Here's how the part is built. I have some questions about the finished solid (model axes, mm). Round coordinates to 2 decimals unless told otherwise and drop trailing zeros. Write each loop counter-clockwise with the first axis right and the second up, starting at its lowest first coordinate (ties: lowest second). Pieces come first, ordered by that corner, then holes. Notation, with made-up numbers: (32, 73.5) -> (38, 73.5) arc R24 cw to (38, 85.5) -> close; hole circle Ø6 at (55, -28.5). An arc over 180 degrees is marked (long way). Answer as CSV lines item,"result".
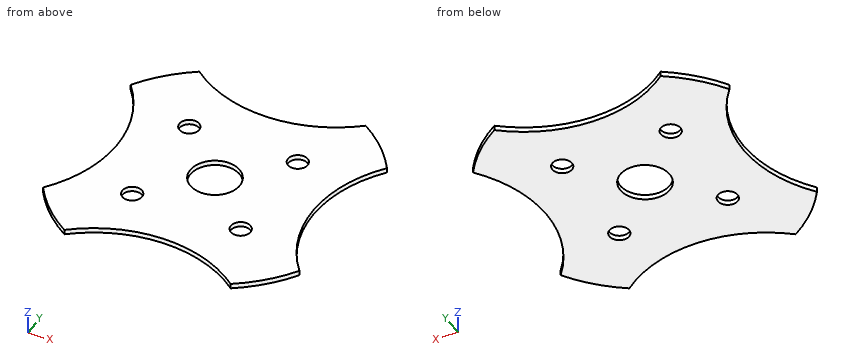
from build123d import *

# Parameters (mm, degrees)
EXTRUDE1_DEPTH     = 3.175
CUT_EXTRUDE1_REACH = 5.175
SKETCH2_R          = 6.35
SKETCH2_R_2        = 15.875


with BuildPart() as part:
    # Sketch1 → Extrude1 (new body)
    with BuildSketch(Plane.XY):
        with BuildLine():
            ThreePointArc((-53.553513238, 82.55), (0, 63.5), (53.553513238, 82.55))
            ThreePointArc((53.553513238, 82.55), (69.579024426, 69.579024426), (82.55, 53.553513238))
            ThreePointArc((82.55, 53.553513238), (63.5, 0), (82.55, -53.553513238))
            ThreePointArc((82.55, -53.553513238), (69.579024426, -69.579024426), (53.553513238, -82.55))
            ThreePointArc((53.553513238, -82.55), (0, -63.5), (-53.553513238, -82.55))
            ThreePointArc((-53.553513238, -82.55), (-69.579024426, -69.579024426), (-82.55, -53.553513238))
            ThreePointArc((-82.55, -53.553513238), (-63.5, 0), (-82.55, 53.553513238))
            ThreePointArc((-82.55, 53.553513238), (-69.579024426, 69.579024426), (-53.553513238, 82.55))
        make_face()
    extrude(amount=-EXTRUDE1_DEPTH)

    # Sketch2 → Cut-Extrude1 (cut, up to next)
    with BuildSketch(Plane(origin=(0, 0, -3.175), x_dir=(-1, 0, 0), z_dir=(0, 0, -1)), mode=Mode.PRIVATE) as cut_extrude1_sk1:
        with Locations((-34.925, 34.925)):
            Circle(SKETCH2_R)
    cut_extrude1_tool1 = extrude(cut_extrude1_sk1.sketch, amount=-CUT_EXTRUDE1_REACH, mode=Mode.PRIVATE) & part.part
    add(cut_extrude1_tool1.solids().sort_by_distance((34.925, 34.925, -3.175))[0], mode=Mode.SUBTRACT)
    # Sketch2 → Cut-Extrude1 (cut, up to next)
    with BuildSketch(Plane(origin=(0, 0, -3.175), x_dir=(-1, 0, 0), z_dir=(0, 0, -1)), mode=Mode.PRIVATE) as cut_extrude1_sk2:
        with Locations((34.925, 34.925)):
            Circle(SKETCH2_R)
    cut_extrude1_tool2 = extrude(cut_extrude1_sk2.sketch, amount=-CUT_EXTRUDE1_REACH, mode=Mode.PRIVATE) & part.part
    add(cut_extrude1_tool2.solids().sort_by_distance((-34.925, 34.925, -3.175))[0], mode=Mode.SUBTRACT)
    # Sketch2 → Cut-Extrude1 (cut, up to next)
    with BuildSketch(Plane(origin=(0, 0, -3.175), x_dir=(-1, 0, 0), z_dir=(0, 0, -1)), mode=Mode.PRIVATE) as cut_extrude1_sk3:
        with Locations((34.925, -34.925)):
            Circle(SKETCH2_R)
    cut_extrude1_tool3 = extrude(cut_extrude1_sk3.sketch, amount=-CUT_EXTRUDE1_REACH, mode=Mode.PRIVATE) & part.part
    add(cut_extrude1_tool3.solids().sort_by_distance((-34.925, -34.925, -3.175))[0], mode=Mode.SUBTRACT)
    # Sketch2 → Cut-Extrude1 (cut, up to next)
    with BuildSketch(Plane(origin=(0, 0, -3.175), x_dir=(-1, 0, 0), z_dir=(0, 0, -1)), mode=Mode.PRIVATE) as cut_extrude1_sk4:
        with Locations((-34.925, -34.925)):
            Circle(SKETCH2_R)
    cut_extrude1_tool4 = extrude(cut_extrude1_sk4.sketch, amount=-CUT_EXTRUDE1_REACH, mode=Mode.PRIVATE) & part.part
    add(cut_extrude1_tool4.solids().sort_by_distance((34.925, -34.925, -3.175))[0], mode=Mode.SUBTRACT)
    # Sketch2 → Cut-Extrude1 (cut, up to next)
    with BuildSketch(Plane(origin=(0, 0, -3.175), x_dir=(-1, 0, 0), z_dir=(0, 0, -1)), mode=Mode.PRIVATE) as cut_extrude1_sk5:
        Circle(SKETCH2_R_2)
    cut_extrude1_tool5 = extrude(cut_extrude1_sk5.sketch, amount=-CUT_EXTRUDE1_REACH, mode=Mode.PRIVATE) & part.part
    add(cut_extrude1_tool5.solids().sort_by_distance((0, 0, -3.175))[0], mode=Mode.SUBTRACT)


solid = part.part
Item 1: Suppose I cut it at B-B, the plane y = 69. List the corners of the cut face in (x, z) for me (3 decimals), then the cut area to 3 significant figures.
Results found:
outline,"(-70.153, -3.175) -> (-30.042, -3.175) -> (-30.042, 0) -> (-70.153, 0) -> close; (30.042, -3.175) -> (70.153, -3.175) -> (70.153, 0) -> (30.042, 0) -> close"
area,"255 mm²"
Item 2: I need wall thicknesses on L1, parallel to Y at x = -0.5, z = -1.2; L2, parallel to X at y = 35, z = -0.5; L3, parallel to X at y = 8, z = -1.15. Which ranges of each line are inside material? Lowest first, please.
Results found:
L1,"y = -63.5 to -15.87, 15.87 to 63.5"
L2,"x = -71.06 to -41.27, -28.58 to 28.58, 41.27 to 71.06"
L3,"x = -63.88 to -13.71, 13.71 to 63.88"
Item 3: Suppose I cut it at C-C, the plane z = -2.4. List the corners of the cut face in (x, y) for me (3 decimals), then the cut area to 3 significant figures.
Results found:
outline,"(-82.55, -53.554) arc R98.4 ccw to (-53.554, -82.55) arc R84.8 cw to (53.554, -82.55) arc R98.4 ccw to (82.55, -53.554) arc R84.8 cw to (82.55, 53.554) arc R98.4 ccw to (53.554, 82.55) arc R84.8 cw to (-53.554, 82.55) arc R98.4 ccw to (-82.55, 53.554) arc R84.8 cw to start; hole circle Ø12.7 at (-34.925, -34.925); hole circle Ø12.7 at (-34.925, 34.925); hole circle Ø31.75 at (0, 0); hole circle Ø12.7 at (34.925, -34.925); hole circle Ø12.7 at (34.925, 34.925)"
area,"18,900 mm²"
Item 4: Suppose I cut it at D-D, the plane y = 39. List the corners of the cut face in (x, z) for me (3 decimals), then the cut area to 3 significant figures.
Results found:
outline,"(-73, -3.175) -> (-39.795, -3.175) -> (-39.795, 0) -> (-73, 0) -> close; (-30.055, -3.175) -> (30.055, -3.175) -> (30.055, 0) -> (-30.055, 0) -> close; (39.795, -3.175) -> (73, -3.175) -> (73, 0) -> (39.795, 0) -> close"
area,"402 mm²"
Item 5: Will these pins go through, and if not, where does the flat tip stop? pin 1 (11.5 mm diameter, centred on x = 34.925, y = 34.925, fed in from -Z); pin 2 (1 mm diameter, centred on x = 38, z = -2, fed in from -Y).
Results found:
pin 1,"passes through"
pin 2,"stops at y = -72.74"
Item 6: Suppose I cut it at A-A, the plane x = 0. List the corners of the cut face in (y, z) for me (3 decimals), then the cut area to 3 significant figures.
Results found:
outline,"(-63.5, -3.175) -> (-15.875, -3.175) -> (-15.875, 0) -> (-63.5, 0) -> close; (15.875, -3.175) -> (63.5, -3.175) -> (63.5, 0) -> (15.875, 0) -> close"
area,"302 mm²"
